Autodesk Inventor part; units mm, degrees
ref_plane "YZ Plane" through (0, 0, 0) normal (1, 0, 0) x (0, 1, 0)
ref_plane "XZ Plane" through (0, 0, 0) normal (0, 1, 0) x (-1, 0, 0)
ref_plane "XY Plane" through (0, 0, 0) normal (0, 0, 1) x (1, 0, 0)
sketch "Skizze1" plane through (0, 0, 0) normal (0, 0, 1) x (1, 0, 0)
  line L0 (-1, 0) -> (-1, 2.5)
  line L1 (-1, 2.5) -> (0, 2.5)
  line L2 (0, 2.5) -> (0, 1.5)
  line L3 (0, 1.5) -> (6, 1.5)
  line L4 (6, 1.5) -> (6, 0)
  line L5 (-1, 0) -> (6, 0)
  line L6 (-4, 0) -> (17, 0)
  line L7 (0, -0.5) -> (0, 3)
  dimension "d0" = 1
  dimension "d1" = 6
  dimension "d2" = 3
  dimension "d3" = 5
revolve "Körper" add sketch "Skizze1" angle 360 about axis through (-1, 0, 0) along (1, 0, 0)
chamfer "Fase1" distance 1 angle 30 1 edges at (6, -1.5, 0) measured on face at (2, 1.4806, -0.2406)
chamfer "Fase2" distance 0.5 angle 45 1 edges at (-1, -2.5, 0) measured on face at (-0.6667, 2.4919, -0.2012)
equation "\"d0\" = KOH"
equation "\"d1\" = NLG"
equation "\"d2\" = NND"
equation "\"d3\" = KOD"
equation "\"d7\" = PHH1"
equation "\"d8\" = FAWI1"
equation "\"d12\" = PHH1"
equation "\"d4\" = PHH2"
equation "\"d6\" = FAWI2"
equation "\"d13\" = PHH2"
equation "\"NLG\" = 6"
equation "\"KOH\" = 1"
equation "\"KOD\" = 5"
equation "\"NND\" = 3"
equation "\"FAWI1\" = 30deg"
equation "\"FAWI2\" = 45deg"
equation "\"PHH2\" = 0.5"
equation "\"PHH1\" = 1"
properties part number "ISO 2341 - A - 3 x 6" material "Stahl"
Source: CAD feature listing. Evaluate the final solid. Frame: model axes, mm. A direction names the side the tool comes from. Round coordinates to 2 decimals unless told otherwise and drop trailing zeros. Write each loop counter-clockwise with the first axis right and the second up, starting at its lowest first coordinate (ties: lowest second). Pieces come first, ordered by that corner, then holes. Notation, with made-up numbers: M 76.5,14.25 L 108.5,14.25 A30 cw 108.5,45.25 Z; hole C 81.5,44 d2. An arc over 180 degrees is marked long. Use CSV: the item, a comma, the result in double quotes. Start each with the question number.
Q1. First-contact query: P1, Ø1.5, axis at y = -1.5, z = -1.5, coming from the +X side. Flat tip, straight axial feed; report the tip coordinate or a pass-through.
Q2. Access query for faces 1 (the face through (0, 2, 0)), 2 (the face through (-0.25, -0.54, -2.44)). Directions: +Z, -Z, +X, -X, +Y, -Y. A direction counts if a zero-diameter tool reaches every point of the face in a straight line with its end or side. Return the directions, or none.
Q3. Cut plane C-C on x = 3.25. Output: boundary loops of the cut face in (y, z), plus the area to 3 significant figures.
Q4. Line query: line 1 (X direction, y = 0.65, z = -1.4); line 2 (Y direction, x = 1.75, z = -0.1); line 3 (Z direction, x = 3.5, y = -0.6). Output: solid intervals per line, ascending. Write a range as from..to.
Q5. Cut plane A-A on y = 0. Output: boundary loops of the cut face in (x, z).
Results found:
1,P1,"x = 5.22"
2,face 1,"+X"
2,face 2,"+X, -X"
3,outline,"C 0,0 d3"
3,area,"7.07 mm^2"
4,line 1,"-1..0"
4,line 2,"-1.5..1.5"
4,line 3,"-1.37..1.37"
5,outline,"M -1,-2 L -0.5,-2.5 L 0,-2.5 L 0,-1.5 L 5,-1.5 L 6,-0.92 L 6,0.92 L 5,1.5 L 0,1.5 L 0,2.5 L -0.5,2.5 L -1,2 Z"
